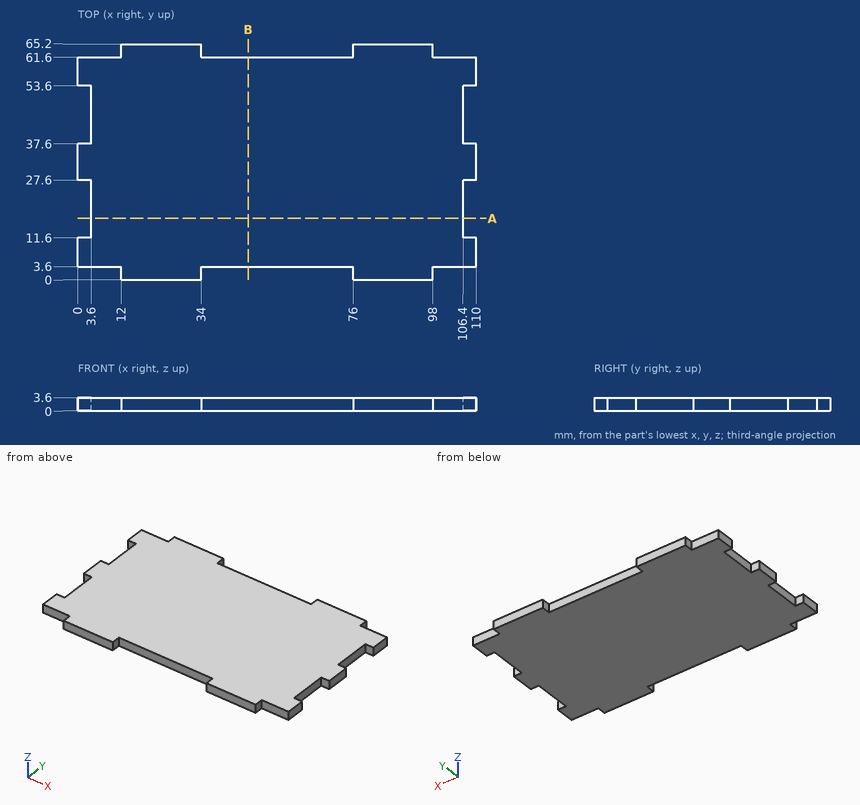
Source: three-view drawing plus pictorial views. Frame: mm from the lowest corner of the part. Give positions to 0.01 mm unless a question says otherwise; leave off trailing zeros. Loops run counter-clockwise (first coordinate to the right, second up) from the corner with the lowest first, then second, coordinate; pieces in that order, holes last. Notation, with made-up numbers: (21, 6) -> (29, 6) arc R26 ccw to (29, 39) -> close; hole circle Ø4 at (37.5, -8.5). An arc over 180 degrees is marked (long way). Use a Markdown table: item, result. Add a question column.
(1) Section query A-A (y = 17). Output: boundary loops of the cut face in (x, z), then the cut area to 3 significant figures.
(2) Section query B-B (x = 47). Output: boundary loops of the cut face in (y, z), then the cut area to 3 significant figures.
(3) Ray query, line 1 (Y direction, x = 45, z = 1.6); line 2 (X direction, y = 39.5, z = 0.4); line 3 (X direction, y = 62.5, z = 2.3). Return the intervals inside material, ascending.
(4) First-contact query: pin 1 Ø1.8 at (x, z) = (1.5, 1.5) entering from -Y; pin 2 Ø1.8 at (y, z) = (43.5, 2) entering from +X; pin 3 Ø1.1 at (y, z) = (2, 1.5) entering from +X; pin 4 Ø10 at (x, y) = (75.5, 11.5) entering from -Z. Flat tips, straight axial feed; report the tip coordinate or a pass-through.
Checked values:
| question | item | result |
|---|---|---|
| 1 | outline | (3.6, 0) -> (106.4, 0) -> (106.4, 3.6) -> (3.6, 3.6) -> close |
| 1 | area | 370 mm^2 |
| 2 | outline | (3.6, 0) -> (61.6, 0) -> (61.6, 3.6) -> (3.6, 3.6) -> close |
| 2 | area | 209 mm^2 |
| 3 | line 1 | 3.6 to 61.6 |
| 3 | line 2 | 3.6 to 106.4 |
| 3 | line 3 | 12 to 34, 76 to 98 |
| 4 | pin 1 | y = 3.6 |
| 4 | pin 2 | x = 106.4 |
| 4 | pin 3 | x = 98 |
| 4 | pin 4 | z = 0 |
